Autodesk Inventor part; units mm, degrees
ref_plane "YZ Plane" through (0, 0, 0) normal (1, 0, 0) x (0, 1, 0)
ref_plane "XZ Plane" through (0, 0, 0) normal (0, 1, 0) x (-1, 0, 0)
ref_plane "XY Plane" through (0, 0, 0) normal (0, 0, 1) x (1, 0, 0)
sketch "Skizze1" plane through (0, 0, 0) normal (0, 0, 1) x (1, 0, 0)
  line L0 (-15, 15) -> (15, 15)
  line L1 (15, 15) -> (15, -15)
  line L2 (15, -15) -> (-15, -15)
  line L3 (-15, 4.8) -> (5.6, 4.8)
  line L4 (5.6, 4.8) -> (5.6, -4.8)
  line L5 (5.6, -4.8) -> (-15, -4.8)
  line L6 (-15, -15) -> (-15, -4.8)
  line L7 (-15, 4.8) -> (-15, 15)
  point P0 (0, 0)
  dimension "d0" = 30
  dimension "d1" = 30
  dimension "d2" = 15
  dimension "d3" = 15
  dimension "d4" = 9.6
  dimension "d5" = 4.8
  dimension "d6" = 5.6
extrude "Extrusion1" add sketch "Skizze1" along normal blind 7
sketch "Skizze2" plane through (0, 0, 0) normal (0, 0, -1) x (-1, 0, 0)
  line L0 (15, -15) -> (-15, -15)
  line L1 (15, -15) -> (-15, -15)
  line L2 (-15, -15) -> (-15, 15)
  line L3 (-15, 15) -> (15, 15)
  line L4 (15, 15) -> (15, -15)
  point P0 (0, 0)
extrude "Extrusion2" add sketch "Skizze2" along normal blind 3
sketch "Skizze3" plane through (0, 0, -3) normal (0, 0, -1) x (-1, 0, 0)
  line L0 (-15, 15) -> (15, 15)
  line L1 (-15, 15) -> (15, 15)
  line L2 (15, 10) -> (15, -10)
  line L3 (15, -15) -> (-15, -15)
  line L4 (15, 15) -> (20, 15)
  line L5 (20, 15) -> (20, 10)
  line L6 (20, 10) -> (15, 10)
  line L7 (-15, 0) -> (15, 0) construction
  line L8 (15, -4.8) -> (15, 4.8)
  line L9 (15, -15) -> (-15, -15)
  line L10 (0, -15) -> (0, 15) construction
  line L11 (15, -15) -> (20, -15)
  line L12 (20, -15) -> (20, -10)
  line L13 (20, -10) -> (15, -10)
  line L14 (-15, 15) -> (-20, 15)
  line L15 (-20, 15) -> (-20, 10)
  line L16 (-20, 10) -> (-15, 10)
  line L17 (-15, -10) -> (-15, 10)
  line L18 (-15, -15) -> (-20, -15)
  line L19 (-20, -15) -> (-20, -10)
  line L20 (-20, -10) -> (-15, -10)
  circle A0 centre (17.5, 12.5) radius 1
  circle A1 centre (17.5, -12.5) radius 1
  circle A2 centre (-17.5, 12.5) radius 1
  circle A3 centre (-17.5, -12.5) radius 1
  point P0 (0, 0)
  point P1 (15, -15)
  point P2 (-15, 15)
  point P3 (-15, -4.8)
  point P4 (-15, 4.8)
  point P5 (-15, -15)
  point P6 (-15, -15)
  dimension "d11" = 5
  dimension "d12" = 5
  dimension "d15" = 2
  dimension "d16" = 2.5
  dimension "d17" = 2.5
extrude "Extrusion3" add sketch "Skizze3" along normal blind 4
properties part number "PotiHalterungUnten"
The model under review builds one solid part; all positions refer to its coordinate system, in mm. A direction names the side the tool comes from. Give positions to 0.01 mm unless a question says otherwise; leave off trailing zeros. Order: outer loops, then holes, each group sorted by start corner. A loop starts at its lowest first (then second) coordinate and runs counter-clockwise, first axis right, second up. Notation, with made-up numbers: M 48.25,7 L 78.25,7 A16 ccw 78.25,30 Z; hole C 77,15 d9. An arc over 180 degrees is marked long. Use one line per item in the form item = value. Start each with the question number.
Item 1: Insertion check: pin 1 Ø4 at (x, y) = (-9.5, -2.5) entering from +Z; pin 2 Ø3 at (x, y) = (-17.5, -12.5) entering from +Z; pin 3 Ø5 at (y, z) = (-10, 2.5) entering from +X. Each pin has a flat end and moves straight along its axis. Give the tip position at first contact, or say it passes through.
Item 2: We need section D-D on z = 2. Give the boundary of the cut face in (x, y), plus the area to 3 significant figures.
Item 3: We need section A-A on y = -12.5. Give the boundary of the cut face in (x, z).
Item 4: For faces 5 (the flat face through (-18, -10, -5)), 6 (the flat face through (-5, 0, 0)), 7 (the flat face through (16, 13, -3)), list the 3-axis set-ups (+Z, -Z, +X, -X, +Y, -Y) from which the entire face can be reached by the end or side of a thin tool; tool diameter is ignored.
Item 5: The part is to be moulded in two halves that separate along Y. For faces 1 (the flat face through (16, -12, -3)), 2 (the flat face through (5.6, 0, 3)), 3 (the flat face through (0, 15, 0)), 4 (the cylindrical face through (16.576, 12.883, -4.972)), say which applies: pulls with the +Y half, pulls with the -Y half, needs draft (parallel to the pull), parting line crosses it, or undercut.
Item 6: To check wall thickness, follow line 1 along Y through (x, z) = (-17.5, -4.85); line 2 along Y through (x, z) = (-1, 6); line 3 along X through (y, z) = (13.5, -0.75). State the ranges of each line that lie inside material, in increasing order. Write a range as from..to.
Item 7: We need section C-C on x = -17.5. Give the boundary of the cut face in (y, z).
Item 8: We need section B-B on x = 16. Give the boundary of the cut face in (y, z), plus the area to 3 significant figures.
Completed:
q1.pin_1 = 0
q1.pin_2 = -3
q1.pin_3 = 15
q2.outline = M -15,-15 L 15,-15 L 15,15 L -15,15 L -15,4.8 L 5.6,4.8 L 5.6,-4.8 L -15,-4.8 Z
q2.area = 702 mm²
q3.outline = M -20,-7 L -18.5,-7 L -18.5,-3 L -20,-3 Z; M -16.5,-7 L 16.5,-7 L 16.5,-3 L 15,-3 L 15,7 L -15,7 L -15,-3 L -16.5,-3 Z; M 18.5,-7 L 20,-7 L 20,-3 L 18.5,-3 Z
q4.face_5 = +Z, -Z, -X
q4.face_6 = +Z, -X
q4.face_7 = +Z, +X, +Y, -Y
q5.face_1 = needs draft
q5.face_2 = undercut
q5.face_3 = pulls with the +Y half
q5.face_4 = undercut
q6.line_1 = -15..-13.5, -11.5..-10, 10..11.5, 13.5..15
q6.line_2 = -15..-4.8, 4.8..15
q6.line_3 = -15..15
q7.outline = M -15,-7 L -13.5,-7 L -13.5,-3 L -15,-3 Z; M -11.5,-7 L -10,-7 L -10,-3 L -11.5,-3 Z; M 10,-7 L 11.5,-7 L 11.5,-3 L 10,-3 Z; M 13.5,-7 L 15,-7 L 15,-3 L 13.5,-3 Z
q8.outline = M -15,-7 L -10,-7 L -10,-3 L -15,-3 Z; M 10,-7 L 15,-7 L 15,-3 L 10,-3 Z
q8.area = 40.0 mm²
